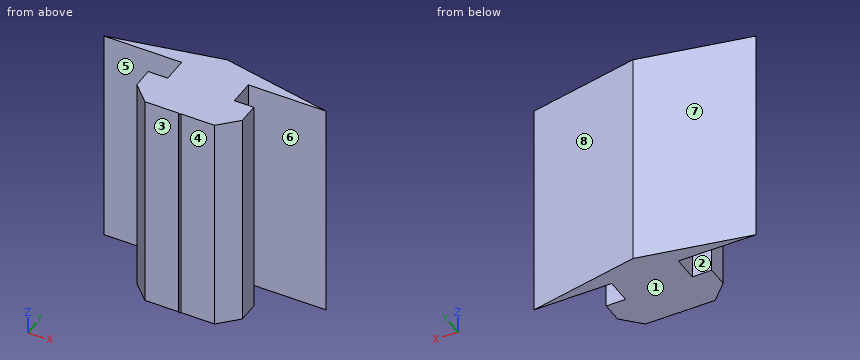
```python
from build123d import *

# Parameters (mm, degrees)
BOSS_EXTRUDE1_DEPTH = 20


with BuildPart() as part:
    # Sketch1 → Boss-Extrude1 (new body)
    with BuildSketch(Plane.XY):
        Polygon((0, 2), (-10, 0), (-4.75, 0), (-3, 0), (0, 0), align=None)
        Polygon((0, 0), (-3, 0), (-3, -1.75), (-3, -1.8), (-3, -2.3), (-4.75, -2.3), (-4.75, -4.189339828), (-3.139339828, -5.8), (-0.1, -5.8), (0, -5.9), (0.1, -5.8), (3.139339828, -5.8), (4.75, -4.189339828), (4.75, -2.3), (3, -2.3), (3, -1.8), (3, -1.75), (3, 0), align=None)
        Polygon((10, 0), (0, 2), (0, 0), (3, 0), (4.75, 0), align=None)
    extrude(amount=BOSS_EXTRUDE1_DEPTH)


solid = part.part
```
Design review of the part built by this model. Coordinates are the model's own, in mm. Face numbers are marked on the shaded views. A direction names the side the tool comes from. Coordinates: 2 decimals unless noted, no trailing zeros. Loops run counter-clockwise (first coordinate to the right, second up) from the corner with the lowest first, then second, coordinate; pieces in that order, holes last.
Q1. We need section B-B on z = 17.5. State the section outline as (x, y) points, and give its area (3 significant figures).
Reported:
outline: (-10, 0) - (-3, 0) - (-3, -2.3) - (-4.75, -2.3) - (-4.75, -4.19) - (-3.14, -5.8) - (-0.1, -5.8) - (0, -5.9) - (0.1, -5.8) - (3.14, -5.8) - (4.75, -4.19) - (4.75, -2.3) - (3, -2.3) - (3, 0) - (10, 0) - (0, 2) - close
area: 64.5 mm2
Q2. Tool access review of the marked faces 4, 5, 6, 7 and 8: name each direction out of +Z, -Z, +X, -X, +Y, -Y from which nothing blocks a thin tool from reaching the whole face with its end or side.
Reported:
face 4: +Z, -Z, +X, -Y
face 5: +Z, -Z, -X
face 6: +Z, -Z, +X
face 7: +Z, -Z, -X, +Y
face 8: +Z, -Z, +X, +Y
Q3. We need section C-C on y = -2. State the section outline as (x, z) points, and give its area (3 significant figures).
Reported:
outline: (-3, 0) - (3, 0) - (3, 20) - (-3, 20) - close
area: 120 mm2
Q4. We need section D-D on x = 5.5. State the section outline as (y, z) points, and give its area (3 significant figures).
Reported:
outline: (0, 0) - (0.9, 0) - (0.9, 20) - (0, 20) - close
area: 18.0 mm2
Q5. To check wall thickness, follow line 1 (X direction, y = -1.75, z = 2); line 2 (X direction, y = -3.5, z = 15.75); line 3 (Y direction, x = 4, z = 16). State the ranges of each line that lie inside material, in increasing order.
Reported:
line 1: x = -3 to 3
line 2: x = -4.75 to 4.75
line 3: y = -4.94 to -2.3, 0 to 1.2
Q6. For pin 1 (3.5 mm diameter, centred on x = 2, z = 12, fed in from -Y); pin 2 (10 mm diameter, centred on x = -0.5, z = 4, fed in from -Y); pin 3 (5.5 mm diameter, centred on x = -6, z = 12.5, fed in from -Y); pin 4 (1.8 mm diameter, centred on y = -1, z = 12.5, fed in from +X), all flat-tipped, find the tip position at first contact; note any pin that passes through.
Reported:
pin 1: stops at y = -5.8
pin 2: stops at y = -5.9
pin 3: stops at y = -5.69
pin 4: stops at x = 3
Q7. The part is to be moulded in two halves that separate along Y. For the marked faces 1, 2 and 3, say which applies: +Y half, -Y half, draft (parallel to the pull), parting line (faces both ways), or undercut.
Reported:
face 1: draft
face 2: undercut
face 3: -Y half
Q8. We need section A-A on x = -3.5. State the section outline as (y, z) points, and give its area (3 significant figures).
Reported:
outline: (-5.44, 0) - (-2.3, 0) - (-2.3, 20) - (-5.44, 20) - close; (0, 0) - (1.3, 0) - (1.3, 20) - (0, 20) - close
area: 88.8 mm2
